Geometry check sheet. Reference: drawing and pictorial views, mm from the part's lowest x, y, z. A direction names the side the tool comes from. Give positions to 0.01 mm unless a question says otherwise; leave off trailing zeros. Order: outer loops, then holes, each group sorted by start corner. A loop starts at its lowest first (then second) coordinate and runs counter-clockwise, first axis right, second up. Notation, with made-up numbers: (9.5, 49) -> (29.5, 49) arc R26 ccw to (29.5, 71) -> close; hole circle Ø4 at (40, 16). An arc over 180 degrees is marked (long way). Write each question's results on one line, items separated by ' | '.
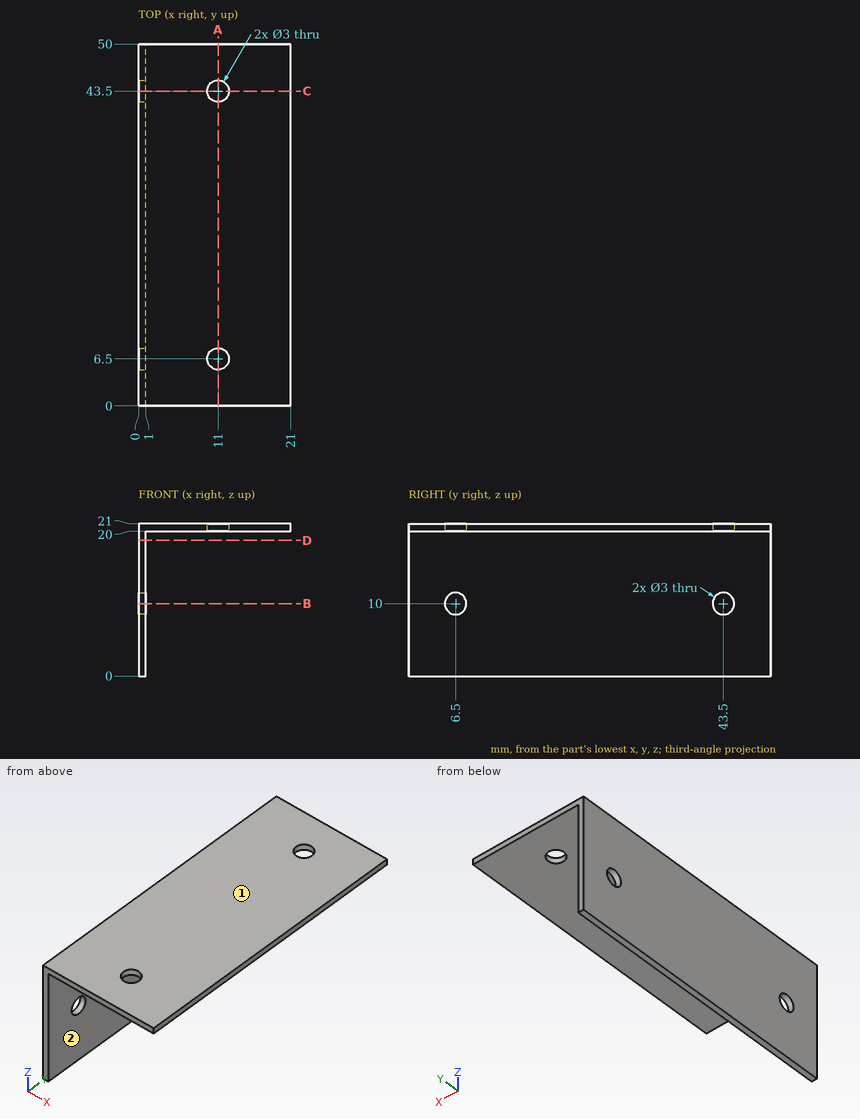
1. Section check A-A on x = 11. Record the cut outline in (y, z).
Verdict:
outline: (0, 20) -> (5, 20) -> (5, 21) -> (0, 21) -> close; (8, 20) -> (42, 20) -> (42, 21) -> (8, 21) -> close; (45, 20) -> (50, 20) -> (50, 21) -> (45, 21) -> close
2. Section check B-B on z = 10. Record the cut outline in (x, y), then the cut area to 3 significant figures.
Verdict:
outline: (0, 0) -> (1, 0) -> (1, 5) -> (0, 5) -> close; (0, 8) -> (1, 8) -> (1, 42) -> (0, 42) -> close; (0, 45) -> (1, 45) -> (1, 50) -> (0, 50) -> close | area: 44.0 mm^2
3. Access from +Z, -Z, +X, -X, +Y, -Y to the whole of each face (thin tool, end or side, straight path). Record for the marked faces 1 and 2.
Verdict:
face 1: +Z, +X, -X, +Y, -Y | face 2: -Z, +X, +Y, -Y
4. Section check C-C on y = 43.5. Record the cut outline in (x, z).
Verdict:
outline: (0, 0) -> (1, 0) -> (1, 8.5) -> (0, 8.5) -> close; (0, 11.5) -> (1, 11.5) -> (1, 20) -> (9.5, 20) -> (9.5, 21) -> (0, 21) -> close; (12.5, 20) -> (21, 20) -> (21, 21) -> (12.5, 21) -> close
5. Material ranges on probe 1 along Y at (x, z) = (11, 20.6); probe 2 along Z at (x, y) = (5.5, 44); probe 3 along X at (y, z) = (21.5, 18), recorded low to high. Write a range as from..to.
Verdict:
probe 1: y = 0..5, 8..42, 45..50 | probe 2: z = 20..21 | probe 3: x = 0..1
6. Gauge pin test, flat ends, axial feed: pin 1 Ø10 at (x, y) = (13.5, 19) entering from -Z; pin 2 Ø1 at (y, z) = (39.5, 9.5) entering from +X. Record the tip position at first contact, or that the pin passes through.
Verdict:
pin 1: stops at z = 20 | pin 2: stops at x = 1
7. Section check D-D on z = 18.75. Record the cut outline in (x, y).
Verdict:
outline: (0, 0) -> (1, 0) -> (1, 50) -> (0, 50) -> close
